Autodesk Inventor part; units mm, degrees
ref_plane "Work Plane1" through (4.699, 0, 1.524) normal (1, 0, 0) x (0, 0, -1)
ref_plane "Work Plane2" through (4.699, 0, 13.4562) normal (0, -1, 0) x (1, 0, 0)
ref_plane "YZ Plane" through (0, 0, 0) normal (1, 0, 0) x (0, 1, 0)
ref_plane "Work Plane1" through (4.699, 0, 1.524) normal (1, 0, 0) x (0, 0, -1)
sketch "Sketch1" plane through (4.699, 0, 1.524) normal (1, 0, 0) x (0, 0, -1)
  line L0 (-11.9322, 40.005) -> (-26.9436, 40.005)
  line L1 (-26.9436, 40.005) -> (-26.9436, 0)
  line L2 (-26.9436, 0) -> (-11.9322, 0)
  line L3 (-11.9322, 0) -> (-11.9322, 40.005)
  circle A0 centre (-19.4379, 20.0025) radius 1.778
  circle A1 centre (-19.4379, 28.0035) radius 1.778
  circle A2 centre (-19.4379, 36.0045) radius 1.778
  line L4 (-11.9322, 20.0025) -> (-25.268, 20.0025)
  circle A3 centre (-19.4379, 12.0015) radius 1.778
  circle A4 centre (-19.4379, 4.0005) radius 1.778
  point P0 (1.524, 0)
  dimension "d0" = 40.005
  dimension "d1" = 15.0114
  dimension "d2" = 3.556
  dimension "d3" = 3.556
  dimension "d4" = 3.556
  dimension "d6" = 8.001
  dimension "d7" = 8.001
extrude "Extrusion1" add sketch "Sketch1" along normal blind 9.398
ref_plane "Work Plane2" through (4.699, 0, 13.4562) normal (0, -1, 0) x (1, 0, 0)
sketch "Sketch2" plane through (4.699, 0, 13.4562) normal (0, -1, 0) x (1, 0, 0)
  line L0 (0, 0) -> (9.398, 0) construction
  line L1 (9.398, 15.0114) -> (9.398, 0) construction
  line L2 (7.874, 13.335) -> (1.524, 13.335)
  line L3 (1.524, 13.335) -> (1.524, 0)
  line L4 (1.524, 0) -> (7.874, 0)
  line L5 (7.874, 0) -> (7.874, 13.335)
  line L6 (0, 0) -> (9.398, 0) construction
  point P0 (-4.699, -13.4562)
  dimension "d10" = 6.35
  dimension "d11" = 1.524
  dimension "d13" = 13.335
extrude "Extrusion2" cut sketch "Sketch2" against normal through all
sketch "Sketch3" plane through (4.699, 0, 28.4676) normal (0, 0, 1) x (1, 0, 0)
  circle A0 centre (4.699, 28.0103) radius 1.778
  circle A1 centre (4.699, 36.0113) radius 1.778
  circle A2 centre (4.699, 20.0093) radius 1.778
  line L0 (0, 18.2245) -> (0, 21.7805) construction
  circle A3 centre (4.699, 11.9947) radius 1.778
  circle A4 centre (4.699, 3.9937) radius 1.778
  point P0 (-4.699, 0)
  dimension "d16" = 3.556
  dimension "d17" = 3.556
  dimension "d19" = 8.001
  dimension "d20" = 8.001
extrude "Extrusion3" cut sketch "Sketch3" against normal through all
fillet "Fillet1" radius 0.635 4 edges at (5.461, 40.005, 13.4562) (5.461, 0, 13.4562) (13.335, 0, 13.4562) (13.335, 40.005, 13.4562)
properties part number "Mini Channel 5 Holes"
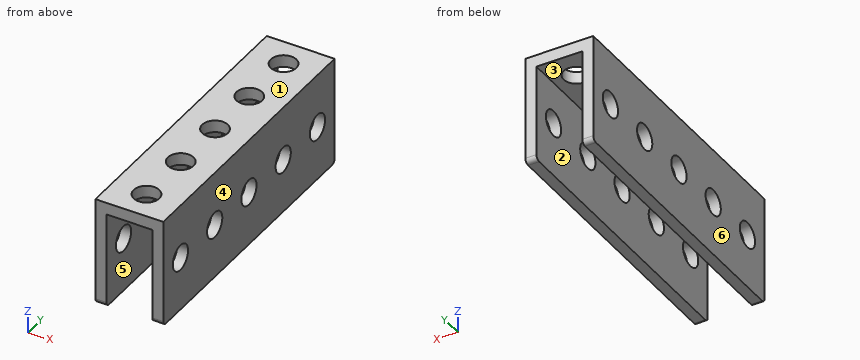
Build history of the part. All positions in model axes, mm. Face numbers are marked on the shaded views. A direction names the side the tool comes from. Round coordinates to 2 decimals unless told otherwise and drop trailing zeros. Loops run counter-clockwise (first coordinate to the right, second up) from the corner with the lowest first, then second, coordinate; pieces in that order, holes last. Notation, with made-up numbers: (-33.5, 62) -> (0.5, 62) arc R18 cw to (0.5, 77) -> close; hole circle Ø8 at (-35, 83.25). An arc over 180 degrees is marked (long way). One line per item, written item: value. Start each with the question number.
Q1. 3-axis set-ups, long thin cutter, end or side, ignore diameter. For the marked faces 5 and 6: which of +Z, -Z, +X, -X, +Y, -Y reach the whole face in a straight line?
Q2. Drop flat-ended pins along their axis: pin 1 Ø2 at (y, z) = (4, 20.96) entering from +X; pin 2 Ø4 at (x, y) = (9.4, 28.01) entering from +Z; pin 3 Ø4 at (x, y) = (9.4, 20.01) entering from -Z. Give the stop position or say it passes through.
Q3. Cut at B-B on y = 19.5. List the corners of the cut face in (x, z), plus the area to 3 significant figures.
Q4. Probe line 1 along X through (y, z) = (18, 16.75); line 2 along X through (y, z) = (36, 27); line 3 along Y through (x, z) = (13, 21) (3 decimals). List the from-to ranges inside material, lowest first.
Q5. Cut at C-C on x = 5.5. List the corners of the cut face in (y, z) (1 decimal), plus the area to 3 significant figures.
Q6. Cut at A-A on z = 25.25. List the corners of the cut face in (x, y) (3 decimals).
Q7. Cut at D-D on x = 10.5. List the corners of the cut face in (y, z) (3 decimals).
Q8. Two-plate mould, pull along X, no slides. Class the marked faces 1, 2, 3 and 4: released by +X, released by -X, zero draft, split by the parting line, or undercut.
Computed:
1. face 5: -Z, +Y, -Y
1. face 6: +Z, -Z, -X, +Y, -Y
2. pin 1: through
2. pin 2: z = 28.47
2. pin 3: z = 26.79
3. outline: (4.7, 13.46) -> (6.22, 13.46) -> (6.22, 19.26) -> (4.7, 19.26) -> close; (4.7, 22.67) -> (6.22, 22.67) -> (6.22, 26.79) -> (7.69, 26.79) -> (7.69, 28.47) -> (4.7, 28.47) -> close; (11.1, 26.79) -> (12.57, 26.79) -> (12.57, 22.67) -> (14.1, 22.67) -> (14.1, 28.47) -> (11.1, 28.47) -> close; (12.57, 13.46) -> (14.1, 13.46) -> (14.1, 19.26) -> (12.57, 19.26) -> close
3. area: 40.3 mm²
4. line 1: 4.7 to 6.22, 12.57 to 14.1
4. line 2: 4.7 to 7.62, 11.18 to 14.1
4. line 3: 0 to 2.223, 5.778 to 10.224, 13.779 to 18.225, 21.78 to 26.226, 29.781 to 34.227, 37.782 to 40.005
5. outline: (0, 14.1) arc R0.6 ccw to (0.6, 13.5) -> (39.4, 13.5) arc R0.6 ccw to (40, 14.1) -> (40, 28.5) -> (0, 28.5) -> close; hole circle Ø3.6 at (4, 21); hole circle Ø3.6 at (12, 21); hole circle Ø3.6 at (20, 21); hole circle Ø3.6 at (28, 21); hole circle Ø3.6 at (36, 21)
5. area: 551 mm²
6. outline: (4.699, 0) -> (6.223, 0) -> (6.223, 40.005) -> (4.699, 40.005) -> close; (12.573, 0) -> (14.097, 0) -> (14.097, 40.005) -> (12.573, 40.005) -> close
7. outline: (0, 26.791) -> (2.598, 26.791) -> (2.598, 28.468) -> (0, 28.468) -> close; (5.389, 26.791) -> (10.599, 26.791) -> (10.599, 28.468) -> (5.389, 28.468) -> close; (13.39, 26.791) -> (18.614, 26.791) -> (18.614, 28.468) -> (13.39, 28.468) -> close; (21.405, 26.791) -> (26.615, 26.791) -> (26.615, 28.468) -> (21.405, 28.468) -> close; (29.406, 26.791) -> (34.616, 26.791) -> (34.616, 28.468) -> (29.406, 28.468) -> close; (37.407, 26.791) -> (40.005, 26.791) -> (40.005, 28.468) -> (37.407, 28.468) -> close
8. face 1: zero draft
8. face 2: undercut
8. face 3: undercut
8. face 4: released by +X
